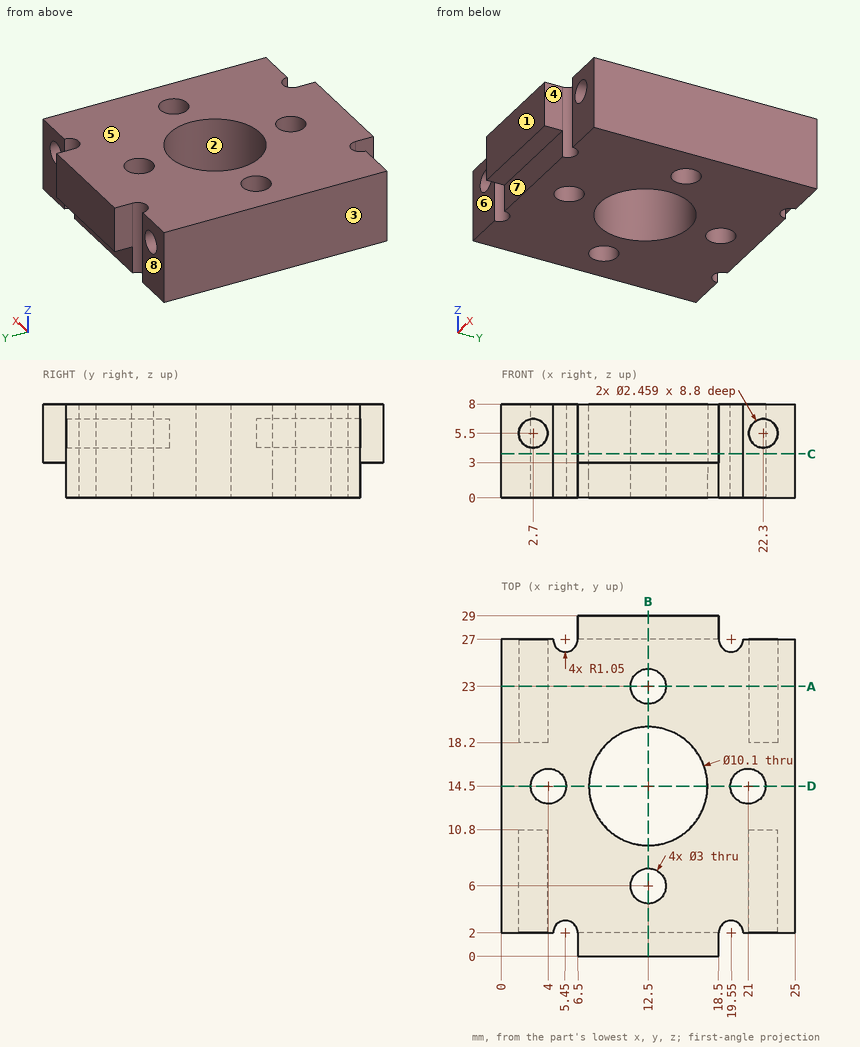
Can you work these out from the drawing? Everything is in mm from the part's minimum corner. A direction names the side the tool comes from. Round coordinates to 2 decimals unless told otherwise and drop trailing zeros. Loops run counter-clockwise (first coordinate to the right, second up) from the corner with the lowest first, then second, coordinate; pieces in that order, holes last. Notation, with made-up numbers: (-17.5, 22.5) - (-6.5, 22.5) arc R13 cw to (-6.5, 46.5) - close; hole circle Ø10 at (-3.75, 6.25). An arc over 180 degrees is marked (long way). One line per question, with ' | ' between items. Start each with the question number.
Q1. I want a section at C-C (z = 3.75). Write out the boundary of the cut face in (x, y).
Q2. We'd pull the mould along X, two halves only. Please class the marked faces 1, 2 and 3: +X half, -X half, draft (parallel to the pull), parting line (faces both ways), or undercut.
Q3. Will these pins go through, and if not, where does the flat tip stop? pin 1 (1.5 mm diameter, centred on x = 21.5, z = 2.5, fed in from +Y); pin 2 (2.5 mm diameter, centred on x = 12.5, y = 23, fed in from +Z); pin 3 (2 mm diameter, centred on x = 22.3, z = 5.5, fed in from -Y); pin 4 (1 mm diameter, centred on y = 0.5, z = 4.5, fed in from -X).
Q4. I want a section at B-B (x = 12.5). Write out the boundary of the cut face in (y, z).
Q5. Please list where these lines run through material, in increasing order: line 1 (Y direction, x = 12.5, z = 2.5); line 2 (Y direction, x = 12.5, z = 6.75); line 3 (Z direction, x = 22.3, y = 5.25). Write a range as [from, to].
Q6. For the marked faces 4, 5, 6, 7 and 8, which set-ups out of +Z, -Z, +X, -X, +Y, -Y let a thin tool reach every point of the face, with its end or its side?
Q7. I want a section at D-D (y = 14.5). Write out the boundary of the cut face in (x, z).
Q8. I want a section at A-A (y = 23). Write out the boundary of the cut face in (x, z).
Response values:
1) outline: (0, 2) - (4.4, 2) arc R1.05 cw to (6.5, 2) - (6.5, 0) - (18.5, 0) - (18.5, 2) arc R1.05 cw to (20.6, 2) - (25, 2) - (25, 27) - (20.6, 27) arc R1.05 cw to (18.5, 27) - (18.5, 29) - (6.5, 29) - (6.5, 27) arc R1.05 cw to (4.4, 27) - (0, 27) - close; hole circle Ø3 at (4, 14.5); hole circle Ø10.1 at (12.5, 14.5); hole circle Ø3 at (12.5, 6); hole circle Ø3 at (12.5, 23); hole circle Ø3 at (21, 14.5)
2) face 1: draft | face 2: undercut | face 3: -X half
3) pin 1: stops at y = 27 | pin 2: passes through | pin 3: stops at y = 10.8 | pin 4: stops at x = 6.5
4) outline: (0, 3) - (2, 3) - (2, 0) - (4.5, 0) - (4.5, 8) - (0, 8) - close; (7.5, 0) - (9.45, 0) - (9.45, 8) - (7.5, 8) - close; (19.55, 0) - (21.5, 0) - (21.5, 8) - (19.55, 8) - close; (24.5, 0) - (27, 0) - (27, 3) - (29, 3) - (29, 8) - (24.5, 8) - close
5) line 1: y = [2, 4.5], [7.5, 9.45], [19.55, 21.5], [24.5, 27] | line 2: y = [0, 4.5], [7.5, 9.45], [19.55, 21.5], [24.5, 29] | line 3: z = [0, 4.27], [6.73, 8]
6) face 4: +Z, -Z, +X, -Y | face 5: +Z, +X, -X, +Y, -Y | face 6: +Z, -Z, -X, -Y | face 7: -Z, +X, -X, -Y | face 8: +Z, -Z, -X, +Y
7) outline: (0, 0) - (2.5, 0) - (2.5, 8) - (0, 8) - close; (5.5, 0) - (7.45, 0) - (7.45, 8) - (5.5, 8) - close; (17.55, 0) - (19.5, 0) - (19.5, 8) - (17.55, 8) - close; (22.5, 0) - (25, 0) - (25, 8) - (22.5, 8) - close
8) outline: (0, 0) - (11, 0) - (11, 8) - (0, 8) - close; (14, 0) - (25, 0) - (25, 8) - (14, 8) - close; hole circle Ø2.46 at (2.7, 5.5); hole circle Ø2.46 at (22.3, 5.5)
